Check sheet for the drawn part. Datum: minimum x, y, z corner. Units: mm. A direction names the side the tool comes from. Give positions to 0.01 mm unless a question says otherwise; leave off trailing zeros. Order: outer loops, then holes, each group sorted by start corner. A loop starts at its lowest first (then second) coordinate and runs counter-clockwise, first axis right, second up.
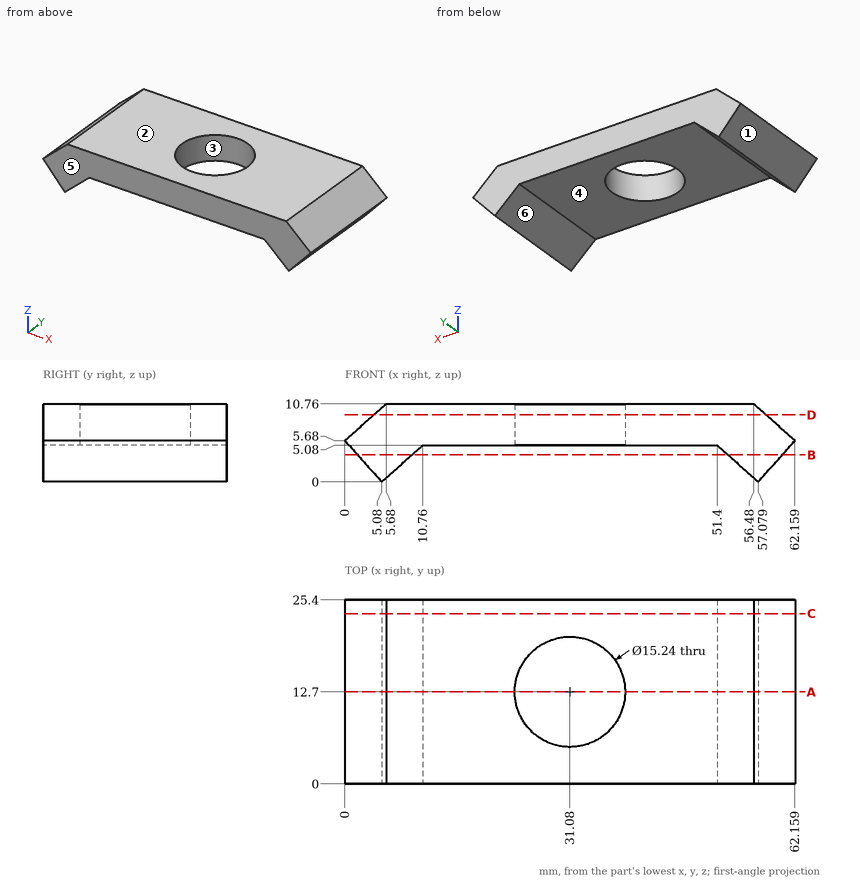
Q1. Go/stop test with flat-tipped pins: P1, Ø2, axis at y = 7, z = 1.5, coming from the -X side (1 decimal); P2, Ø2, axis at y = 4, z = 7.5, coming from the +X side; P3, Ø1, axis at y = 8, z = 8, coming from the +X side (1 decimal); P4, Ø5, axis at x = 45.5, z = 8, coming from the -Y side. Record where each tip stops, or that it passes through.
Q2. Draft check along X on the marked faces 1, 2, 3 and 4. Enter one of: pulls with the +X half, pulls with the -X half, needs draft (parallel to the pull), parting line crosses it, or undercut.
Q3. Sectioned sample at A-A, the plane y = 12.7. Record the cut outline in (x, z), plus the area to 3 significant figures.
Q4. Sectioned sample at B-B, the plane z = 3.75. Record the cut outline in (x, y), plus the area to 3 significant figures.
Q5. Material ranges on line 1 (Z direction, x = 17.5, y = 14.5); line 2 (X direction, y = 16.5, z = 1.75) (1 decimal); line 3 (X direction, y = 1.75, z = 3) (1 decimal), recorded low to high.
Q6. Tool access check on the marked faces 5 and 6. Record the directions out of +Z, -Z, +X, -X, +Y, -Y that give a thin tool (end or side, any length) a straight path to the whole face; none if there is none.
Q7. Sectioned sample at C-C, the plane y = 23.5. Record the cut outline in (x, z), plus the area to 3 significant figures.
Q8. Sectioned sample at D-D, the plane z = 9.25. Record the cut outline in (x, y), plus the area to 3 significant figures.
Filled in:
1. P1: stops at x = 2.8
1. P2: stops at x = 61.24
1. P3: stops at x = 60.1
1. P4: stops at y = 0
2. face 1: pulls with the -X half
2. face 2: needs draft
2. face 3: undercut
2. face 4: undercut
3. outline: (0, 5.68) - (5.08, 0) - (10.76, 5.08) - (23.46, 5.08) - (23.46, 10.76) - (5.68, 10.76) - close; (38.7, 5.08) - (51.4, 5.08) - (57.08, 0) - (62.16, 5.68) - (56.48, 10.76) - (38.7, 10.76) - close
3. area: 289 mm2
4. outline: (1.73, 0) - (9.27, 0) - (9.27, 25.4) - (1.73, 25.4) - close; (52.89, 0) - (60.43, 0) - (60.43, 25.4) - (52.89, 25.4) - close
4. area: 383 mm2
5. line 1: z = 5.08 to 10.76
5. line 2: x = 3.5 to 7, 55.1 to 58.6
5. line 3: x = 2.4 to 8.4, 53.7 to 59.8
6. face 5: +Z, -Z, +X, -X, -Y
6. face 6: -Z, +Y, -Y
7. outline: (0, 5.68) - (5.08, 0) - (10.76, 5.08) - (51.4, 5.08) - (57.08, 0) - (62.16, 5.68) - (56.48, 10.76) - (5.68, 10.76) - close
7. area: 376 mm2
8. outline: (3.99, 0) - (58.17, 0) - (58.17, 25.4) - (3.99, 25.4) - close; hole circle Ø15.24 at (31.08, 12.7)
8. area: 1,190 mm2
